Can you work these out from the model? Positions are in its coordinate system, mm. Face numbers are marked on the shaded views. A direction names the side the tool comes from. Coordinates: 2 decimals unless noted, no trailing zeros. Order: outer loops, then holes, each group sorted by start corner. A loop starts at its lowest first (then second) coordinate and runs counter-clockwise, first axis right, second up. Notation, with made-up numbers: M 79,-7.75 L 102,-7.75 A24 cw 102,10.25 Z; hole C -30.5,-33.5 d6. An arc over 180 degrees is marked long. Answer as a JSON object with one key per item and string values.
from build123d import *

# Parameters (mm, degrees)
SKETCH_1_W          = 35
SKETCH_1_H          = 24
EXTRUDE_1_DEPTH     = 7
SKETCH_2_W          = 31.5
SKETCH_2_H          = 20.5
CUT_EXTRUDE_1_DEPTH = 3
SKETCH_3_W          = 28
SKETCH_3_H          = 17
CUT_EXTRUDE_2_DEPTH = 2
EXTRUDE_2_DEPTH     = 17
SKETCH_6_W          = 33
SKETCH_6_H          = 6
CUT_EXTRUDE_3_DEPTH = 3.5


with BuildPart() as part:
    # 草图1 → 凸台-拉伸1 (new body)
    with BuildSketch(Plane.XY):
        Rectangle(SKETCH_1_W, SKETCH_1_H)
    extrude(amount=EXTRUDE_1_DEPTH)

    # 草图2 → 切除-拉伸1 (cut)
    with BuildSketch(Plane.XY.offset(7)):
        Rectangle(SKETCH_2_W, SKETCH_2_H)
    extrude(amount=-CUT_EXTRUDE_1_DEPTH, mode=Mode.SUBTRACT)

    # 草图3 → 切除-拉伸2 (cut)
    with BuildSketch(Plane.XY.offset(4)):
        Rectangle(SKETCH_3_W, SKETCH_3_H)
    extrude(amount=-CUT_EXTRUDE_2_DEPTH, mode=Mode.SUBTRACT)

    # 草图4 → 凸台-拉伸2 (add)
    with BuildSketch(Plane.XZ.offset(-8.5)):
        with BuildLine():
            Line((-15, 3), (-15, 1))
            Line((-15, 1), (15, 1))
            Line((15, 1), (15, 3))
            Line((15, 3), (14, 3))
            ThreePointArc((14, 3), (13.3, 3.7), (12.6, 3))
            ThreePointArc((12.6, 3), (11.9, 2.3), (11.2, 3))
            ThreePointArc((11.2, 3), (10.5, 3.7), (9.8, 3))
            ThreePointArc((9.8, 3), (9.1, 2.3), (8.4, 3))
            ThreePointArc((8.4, 3), (7.7, 3.7), (7, 3))
            ThreePointArc((7, 3), (6.3, 2.3), (5.6, 3))
            ThreePointArc((5.6, 3), (4.9, 3.7), (4.2, 3))
            ThreePointArc((4.2, 3), (3.5, 2.3), (2.8, 3))
            ThreePointArc((2.8, 3), (2.1, 3.7), (1.4, 3))
            ThreePointArc((1.4, 3), (0.7, 2.3), (0, 3))
            ThreePointArc((0, 3), (-0.7, 3.7), (-1.4, 3))
            ThreePointArc((-1.4, 3), (-2.1, 2.3), (-2.8, 3))
            ThreePointArc((-2.8, 3), (-3.5, 3.7), (-4.2, 3))
            ThreePointArc((-4.2, 3), (-4.9, 2.3), (-5.6, 3))
            ThreePointArc((-5.6, 3), (-6.3, 3.7), (-7, 3))
            ThreePointArc((-7, 3), (-7.7, 2.3), (-8.4, 3))
            ThreePointArc((-8.4, 3), (-9.1, 3.7), (-9.8, 3))
            ThreePointArc((-9.8, 3), (-10.5, 2.3), (-11.2, 3))
            ThreePointArc((-11.2, 3), (-11.9, 3.7), (-12.6, 3))
            ThreePointArc((-12.6, 3), (-13.3, 2.3), (-14, 3))
            Line((-14, 3), (-15, 3))
        make_face()
    extrude(amount=EXTRUDE_2_DEPTH)

    # 草图6 → 切除-拉伸3 (cut)
    with BuildSketch(Plane.XZ.offset(12)):
        with Locations((0, 4)):
            Rectangle(SKETCH_6_W, SKETCH_6_H)
    extrude(amount=-CUT_EXTRUDE_3_DEPTH, mode=Mode.SUBTRACT)


solid = part.part
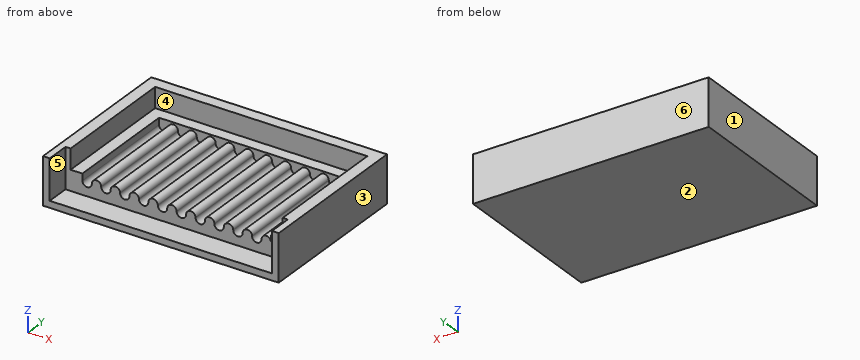
Item 1: I want a section at B-B, the plane z = 1.5. Write out the boundary of the cut face in (x, y), plus the area to 4 significant figures.
Answers follow:
{"outline": "M -17.5,-12 L -16.5,-12 L -16.5,-8.5 L 16.5,-8.5 L 16.5,-12 L 17.5,-12 L 17.5,12 L -17.5,12 Z", "area": "724.5 mm^2"}
Item 2: Please list where these lines run through material, in increasing order: line 1 (X direction, y = 1.25, z = 3.75); line 2 (X direction, y = -1, z = 5.5); line 3 (Y direction, x = -8, z = 5).
Answers follow:
{"line 1": "x = -17.5 to -14, 14 to 17.5", "line 2": "x = -17.5 to -15.75, 15.75 to 17.5", "line 3": "y = 10.25 to 12"}
Item 3: I want a section at D-D, the plane x = -10.5. Write out the boundary of the cut face in (y, z), plus the area to 4 significant figures.
Answers follow:
{"outline": "M -12,0 L 12,0 L 12,7 L 10.25,7 L 10.25,4 L 8.5,4 L 8.5,2.3 L -8.5,2.3 L -8.5,1 L -12,1 Z", "area": "61.85 mm^2"}
Item 4: I'm going to push flat-ended pins straight in: pin 1 (1 mm diameter, centred on x = 0, y = -10.5, fed in from +Z); pin 2 (1.5 mm diameter, centred on x = -2.5, y = 6, fed in from +Z); pin 3 (1.4 mm diameter, centred on x = 1.5, z = 3.5, fed in from -Y). Where does each tip first touch, or does it pass through?
Answers follow:
{"pin 1": "stops at z = 1", "pin 2": "stops at z = 3.65", "pin 3": "stops at y = -8.5"}
Item 5: Which directions (+Z, -Z, +X, -X, +Y, -Y) give clear straight access to the entire face, cutting with the end or side of a thin tool? Please do the marked faces 5 and 6.
Answers follow:
{"face 5": "+Z, -Y", "face 6": "+Z, -Z, +X, -X, +Y"}
Item 6: If we mould it in two halves opening along X, with no side actions, what happens to the marked faces 1, 2, 3 and 4? For each: pulls with the +X half, pulls with the -X half, needs draft (parallel to the pull), parting line crosses it, or undercut.
Answers follow:
{"face 1": "pulls with the -X half", "face 2": "needs draft", "face 3": "pulls with the +X half", "face 4": "undercut"}
Item 7: I want a section at A-A, the plane x = -15. Write out the boundary of the cut face in (y, z), plus the area to 4 significant figures.
Answers follow:
{"outline": "M -12,0 L 12,0 L 12,7 L 10.25,7 L 10.25,4 L -8.5,4 L -8.5,1 L -12,1 Z", "area": "90.75 mm^2"}
